```python
from build123d import *

# Parameters (mm, degrees)
SKETCH_1_R          = 2.025
EXTRUDE_1_DEPTH     = 2.1
CUT_EXTRUDE_1_DEPTH = 21.1
FILLET_1_R          = 1.1


with BuildPart() as part:
    # 草图1 → 凸台-拉伸1 (new body)
    with BuildSketch(Plane.XY):
        with BuildLine():
            Line((-12, 16.525), (12, 16.525))
            ThreePointArc((12, 16.525), (15.406694788, 14.643608085), (15.628630306, 10.758257453))
            Line((15.628630306, 10.758257453), (3.628630306, -14.241742547))
            ThreePointArc((3.628630306, -14.241742547), (0, -16.525), (-3.628630306, -14.241742547))
            Line((-3.628630306, -14.241742547), (-15.628630306, 10.758257453))
            ThreePointArc((-15.628630306, 10.758257453), (-15.406694788, 14.643608085), (-12, 16.525))
        make_face()
        with Locations((-12, 12.5)):
            Circle(SKETCH_1_R, mode=Mode.SUBTRACT)
        with Locations((12, 12.5)):
            Circle(SKETCH_1_R, mode=Mode.SUBTRACT)
        with Locations((0, -12.5)):
            Circle(SKETCH_1_R, mode=Mode.SUBTRACT)
    extrude(amount=EXTRUDE_1_DEPTH)

    # 草图2 → 切除-拉伸1 (cut)
    with BuildSketch(Plane.XY.offset(2.1)):
        Polygon((-8.861262909, 10.525), (0, -7.935964395), (8.861262909, 10.525), align=None)
    extrude(amount=-CUT_EXTRUDE_1_DEPTH, mode=Mode.SUBTRACT)

    # 圆角1
    fillet_1_edges = [part.edges().sort_by_distance(p)[0] for p in [
        (-8.861262909, 10.525, 1.05),
        (8.861262909, 10.525, 1.05),
        (0, -7.935964395, 1.05),
    ]]
    fillet(fillet_1_edges, radius=FILLET_1_R)


solid = part.part
```
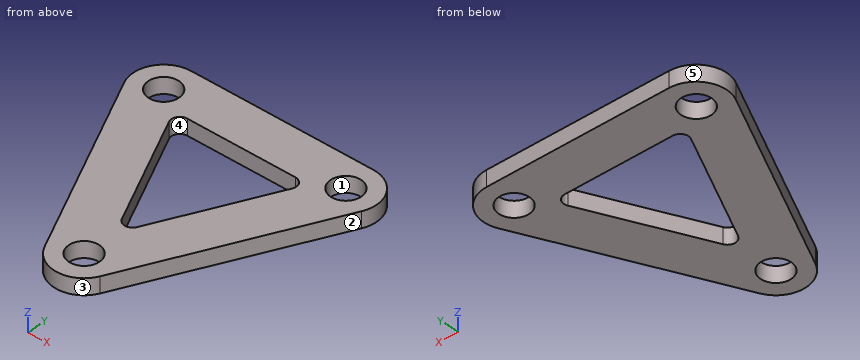
Verification items for the finished model (mm, model axes). Face numbers are marked on the shaded views. A direction names the side the tool comes from. Give positions to 0.01 mm unless a question says otherwise; leave off trailing zeros. Order: outer loops, then holes, each group sorted by start corner. A loop starts at its lowest first (then second) coordinate and runs counter-clockwise, first axis right, second up. Notation, with made-up numbers: M 74.25,80.25 L 132.25,80.25 A18 ccw 132.25,93.25 Z; hole C 23.25,89.5 d10. An arc over 180 degrees is marked long. Answer in a Markdown table with one row per item. Add a question column.
Item 1: Section check B-B, the plane y = -12. Enter the section's corners in (x, z), and give its area (3 significant figures).
Item 2: Tool access check on the marked faces 4 and 5. Record the directions out of +Z, -Z, +X, -X, +Y, -Y that give a thin tool (end or side, any length) a straight path to the whole face; none if there is none.
Item 3: Mould release check, pull along X, two halves, no side actions. Record for the marked faces 1, 2 and 3: released by +X, released by -X, zero draft, split by the parting line, or undercut.
Item 4: Gauge pin test, flat end, axial feed: pin 1 (0.6 mm diameter, centred on x = 3, z = 1.5, fed in from -Y). Record the tip position at first contact, or that the pin passes through.
Item 5: Scan lines: probe 1 along X at (y, z) = (11, 0.15); probe 2 along Y at (x, z) = (0, 1.15) (3 decimals); probe 3 along X at (y, z) = (0.5, 1.6). Record each from-to range of solid material in increasing order. Write a range as from..to.
Item 6: Section check D-D, the plane y = 0. Enter the section's corners in (x, z).
Item 7: Section check A-A, the plane x = 0. Enter the section's corners in (y, z) (3 decimals).
Item 8: Section check C-C, the plane z = 0.4. Enter the section's corners in (x, y) (3 decimals).
Filled sheet:
| question | item | result |
|---|---|---|
| 1 | outline | M -4.7,0 L -1.96,0 L -1.96,2.1 L -4.7,2.1 Z; M 1.96,0 L 4.7,0 L 4.7,2.1 L 1.96,2.1 Z |
| 1 | area | 11.5 mm^2 |
| 2 | face 4 | +Z, -Z |
| 2 | face 5 | +Z, -Z, -X |
| 3 | face 1 | undercut |
| 3 | face 2 | released by +X |
| 3 | face 3 | split by the parting line |
| 4 | pin 1 | stops at y = -15.49 |
| 5 | probe 1 | x = -15.74..-13.36, -10.64..10.64, 13.36..15.74 |
| 5 | probe 2 | y = -16.525..-14.525, -10.475..-6.494, 10.525..16.525 |
| 5 | probe 3 | x = -10.7..-4.05, 4.05..10.7 |
| 6 | outline | M -10.46,0 L -3.81,0 L -3.81,2.1 L -10.46,2.1 Z; M 3.81,0 L 10.46,0 L 10.46,2.1 L 3.81,2.1 Z |
| 7 | outline | M -16.525,0 L -14.525,0 L -14.525,2.1 L -16.525,2.1 Z; M -10.475,0 L -6.494,0 L -6.494,2.1 L -10.475,2.1 Z; M 10.525,0 L 16.525,0 L 16.525,2.1 L 10.525,2.1 Z |
| 8 | outline | M -15.629,10.758 L -3.629,-14.242 A4.025 ccw 3.629,-14.242 L 15.629,10.758 A4.025 ccw 12,16.525 L -12,16.525 A4.025 ccw Z; hole C -12,12.5 d4.05; hole M -8.105,8.949 L -0.992,-5.87 A1.1 ccw 0.992,-5.87 L 8.105,8.949 A1.1 ccw 7.113,10.525 L -7.113,10.525 A1.1 ccw Z; hole C 0,-12.5 d4.05; hole C 12,12.5 d4.05 |
